from build123d import *

# Parameters (mm, degrees)
SKETCH1_W                      = 150
SKETCH1_H                      = 230
BASE_FLANGE1_DEPTH             = 2
EDGE_FLANGE1_STRIP_W           = 28
EDGE_FLANGE1_STRIP_H           = 2
EDGE_FLANGE1_STRIP_CUT_DEPTH   = 230
EDGE_FLANGE1_STRIP_2_W         = 28
EDGE_FLANGE1_STRIP_2_H         = 2
EDGE_FLANGE1_STRIP_CUT_2_DEPTH = 230
EDGE_FLANGE1_DEPTH             = 230
EDGE_FLANGE1_BEND_DEPTH        = 230
SKETCH15_OUTSIDE_W             = 298.254
SKETCH15_OUTSIDE_H             = 250.254
SKETCH15_OUTSIDE_R             = 8
CUT_EXTRUDE1_DEPTH             = 264.326793168
SKETCH16_R                     = 8
CUT_EXTRUDE2_DEPTH             = 228.055059487
CUT_EXTRUDE3_DEPTH             = 228.055059487
SKETCHED_START                 = 47
SKETCHED_BEND1_DEPTH           = 11.052994728
SKETCHED_BEND1_2_DEPTH         = 11.052994728
CUT_EXTRUDE4_REACH             = 241.866
SKETCH20_R                     = 1.25


# Read off the part's stored shape, not the designer's step: Sketched Bend1
# Sheet-metal steps are written as plain solids
with BuildPart() as part:
    # Sketch1 → Base-Flange1 (new body)
    with BuildSketch(Plane(origin=(0, 0, 0), x_dir=(1, 0, 0), z_dir=(0, 1, 0))):
        Rectangle(SKETCH1_W, SKETCH1_H)
    extrude(amount=-BASE_FLANGE1_DEPTH)

    # Edge-Flange1 strip (across the edge) → Edge-Flange1 strip cut (cut)
    with BuildSketch(Plane(origin=(75, 0, 115), x_dir=(-1, 0, 0), z_dir=(0, 0, -1))):
        with Locations((-4, -1)):
            Rectangle(EDGE_FLANGE1_STRIP_W, EDGE_FLANGE1_STRIP_H)
    extrude(amount=EDGE_FLANGE1_STRIP_CUT_DEPTH, mode=Mode.SUBTRACT)

    # Edge-Flange1 strip 2 (across the edge) → Edge-Flange1 strip cut 2 (cut)
    with BuildSketch(Plane(origin=(-75, 0, -115), x_dir=(1, 0, 0), z_dir=(0, 0, 1))):
        with Locations((-4, -1)):
            Rectangle(EDGE_FLANGE1_STRIP_2_W, EDGE_FLANGE1_STRIP_2_H)
    extrude(amount=EDGE_FLANGE1_STRIP_CUT_2_DEPTH, mode=Mode.SUBTRACT)

    # Edge-Flange1 section (across the edge) → Edge-Flange1 (add)
    with BuildSketch(Plane(origin=(75, 0, 115), x_dir=(-1, 0, 0), z_dir=(0, 0, -1))):
        with BuildLine():
            Line((-2, 10), (-2, 180))
            Line((-2, 180), (0, 180))
            Line((0, 180), (0, 10))
            ThreePointArc((0, 10), (2.928932188, 2.928932188), (10, 0))
            Line((10, 0), (10, -2))
            ThreePointArc((10, -2), (1.514718626, 1.514718626), (-2, 10))
        make_face()
    extrude(amount=EDGE_FLANGE1_DEPTH)

    # Edge-Flange1 section 2 (across the edge) → Edge-Flange1 bend (add)
    with BuildSketch(Plane(origin=(-75, 0, -115), x_dir=(1, 0, 0), z_dir=(0, 0, 1))):
        with BuildLine():
            Line((-2, 10), (-2, 180))
            Line((-2, 180), (0, 180))
            Line((0, 180), (0, 10))
            ThreePointArc((0, 10), (2.928932188, 2.928932188), (10, 0))
            Line((10, 0), (10, -2))
            ThreePointArc((10, -2), (1.514718626, 1.514718626), (-2, 10))
        make_face()
    extrude(amount=EDGE_FLANGE1_BEND_DEPTH)

    # Sketch15 outside → Cut-Extrude1 (cut, through all)
    # profile 1 of 4: a face of its own
    with BuildSketch(Plane.ZY.offset(77)):
        with Locations((0, 89)):
            Rectangle(SKETCH15_OUTSIDE_W, SKETCH15_OUTSIDE_H)
        with BuildLine():
            Line((21.083470393, 171.180744276), (96.507242037, 119.243178795))
            ThreePointArc((96.507242037, 119.243178795), (101.277963521, 113.867184852), (103, 106.888955512))
            Line((103, 106.888955512), (103, 16))
            ThreePointArc((103, 16), (104.757359313, 11.757359313), (109, 10))
            Line((109, 10), (110, 10))
            ThreePointArc((110, 10), (113.535533906, 8.535533906), (115, 5))
            Line((115, 5), (115, -2))
            Line((115, -2), (-115, -2))
            Line((-115, -2), (-115, 99))
            Line((-115, 99), (-115, 150))
            ThreePointArc((-115, 150), (-106.213203436, 171.213203436), (-85, 180))
            Line((-85, 180), (-7.274003064, 180))
            ThreePointArc((-7.274003064, 180), (7.574612801, 177.744304445), (21.083470393, 171.180744276))
        make_face(mode=Mode.SUBTRACT)
    # profile 2 of 4: a face of its own
    with BuildSketch(Plane.ZY.offset(77)):
        with Locations(Location((50, 93, 0), (0, 0, 270))):
            Circle(SKETCH15_OUTSIDE_R)
    # profile 3 of 4: a face of its own
    with BuildSketch(Plane.ZY.offset(77)):
        with Locations(Location((-85, 150, 0), (0, 0, 270))):
            Circle(SKETCH15_OUTSIDE_R)
    # profile 4 of 4: a face of its own
    with BuildSketch(Plane.ZY.offset(77)):
        with Locations(Location((-10, 65, 0), (0, 0, 270))):
            Circle(SKETCH15_OUTSIDE_R)
    extrude(amount=-CUT_EXTRUDE1_DEPTH, mode=Mode.SUBTRACT)

    # Sketch16 → Cut-Extrude2 (cut, through all)
    with BuildSketch(Plane(origin=(0, 0, 0), x_dir=(1, 0, 0), z_dir=(0, 1, 0))):
        with Locations(Location((-42, 39, 0), (0, 0, 270))):
            Circle(SKETCH16_R)
        with Locations(Location((42, 39, 0), (0, 0, 90))):
            Circle(SKETCH16_R)
        with Locations(Location((-42, -31, 0), (0, 0, 90))):
            Circle(SKETCH16_R)
        with Locations(Location((42, -31, 0), (0, 0, 270))):
            Circle(SKETCH16_R)
        with BuildLine():
            Line((7.5, 20), (7.5, -20))
            ThreePointArc((7.5, -20), (0, -27.5), (-7.5, -20))
            Line((-7.5, -20), (-7.5, 20))
            ThreePointArc((-7.5, 20), (0, 27.5), (7.5, 20))
        make_face()
    extrude(amount=-CUT_EXTRUDE2_DEPTH, mode=Mode.SUBTRACT)

    # Sketch18 → Cut-Extrude3 (cut, through all)
    with BuildSketch(Plane(origin=(0, 0, 0), x_dir=(1, 0, 0), z_dir=(0, 1, 0))):
        Polygon((31.4, -45), (44.4, -45), (44.4, -60.052994728), (31.4, -60.052994728), (31.4, -58.052994728), (42.4, -58.052994728), (42.4, -47), (31.4, -47), align=None)
    extrude(amount=-CUT_EXTRUDE3_DEPTH, mode=Mode.SUBTRACT)

    # Sketched Bend1 outline → Sketched Bend1 (cut)
    with BuildSketch(Plane.XY.offset(SKETCHED_START)):
        with BuildLine():
            ThreePointArc((34.035602398, 0), (33.054267209, -1.443395312), (31.4, -2))
            Line((31.4, -2), (42.4, -2))
            Line((42.4, -2), (42.4, 0))
            Line((42.4, 0), (34.035602398, 0))
        make_face()
    extrude(amount=SKETCHED_BEND1_DEPTH, mode=Mode.SUBTRACT)

    # Sketched Bend1 2 outline → Sketched Bend1 2 (add)
    with BuildSketch(Plane.XY.offset(SKETCHED_START)):
        with BuildLine():
            Line((31.4, 0), (34.035602398, 0))
            ThreePointArc((34.035602398, 0), (34.111233029, 0.364854094), (34.1366, 0.7366))
            Line((34.1366, 0.7366), (34.1366, 9.008755099))
            Line((34.1366, 9.008755099), (32.1366, 9.008755099))
            Line((32.1366, 9.008755099), (32.1366, 0.7366))
            ThreePointArc((32.1366, 0.7366), (31.920854855, 0.215745145), (31.4, 0))
        make_face()
    extrude(amount=SKETCHED_BEND1_2_DEPTH)

    # Sketch20 → Cut-Extrude4 (cut, up to next)
    with BuildSketch(Plane.ZY.offset(-32.1366), mode=Mode.PRIVATE) as cut_extrude4_sk1:
        with Locations(Location((52.526497364, 4.9366, 0), (0, 0, 270))):
            Circle(SKETCH20_R)
    cut_extrude4_tool1 = extrude(cut_extrude4_sk1.sketch, amount=-CUT_EXTRUDE4_REACH, mode=Mode.PRIVATE) & part.part
    add(cut_extrude4_tool1.solids().sort_by_distance((32.1366, 4.9366, 52.526497))[0], mode=Mode.SUBTRACT)


solid = part.part
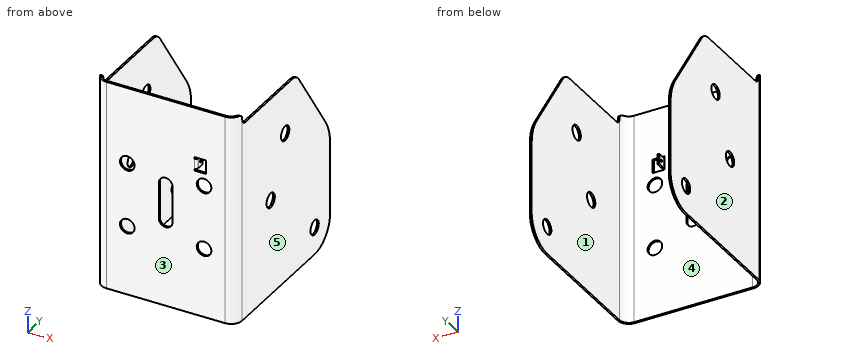
Geometry: final body of the model. Coordinates: model frame, mm. Face numbers are marked on the shaded views. A direction names the side the tool comes from. Coordinates: 2 decimals unless noted, no trailing zeros. Loops run counter-clockwise (first coordinate to the right, second up) from the corner with the lowest first, then second, coordinate; pieces in that order, holes last. Notation, with made-up numbers: (82.25, 59) - (96.25, 59) arc R21 cw to (96.25, 90) - close; hole circle Ø6 at (78, 88). An arc over 180 degrees is marked (long way). One line per question, with ' | ' between items. Start each with the question number.
(1) Cut plane D-D on z = -10. Output: boundary loops of the cut face in (x, y), and give its area (3 significant figures).
(2) First-contact query: pin 1 (1.6 mm diameter, centred on y = -1, z = 50.5, fed in from -X); pin 2 (3 mm diameter, centred on y = 4.94, z = 52.53, fed in from +X); pin 3 (10 mm diameter, centred on x = -53, z = -14, fed in from +Y); pin 4 (21 mm diameter, centred on x = 42, z = -39, fed in from -Y). Flat tips, straight axial feed; report the tip coordinate or a pass-through.
(3) Draft query along X for the marked faces 3, 4 and 5. Return one class per face: +X half, -X half, draft (parallel to the pull), parting line (faces both ways), or undercut.
(4) Cut plane C-C on z = -39. Output: boundary loops of the cut face in (x, y), and give its area (3 significant figures).
(5) Cut plane A-A on x = -42. Output: boundary loops of the cut face in (y, z).
(6) Reachability of the marked faces 1 and 2 from +Z, -Z, +X, -X, +Y, -Y: full face, straight path, thin tool, end or side. Return the list, or none.
(7) Ray query, L1, parallel to X at y = 24, z = 55.5; L2, parallel to X at y = -1, z = 31; L3, parallel to Z at x = -76.05, y = 93. Return the intervals inside material, ascending. Write a range as from..to.
(8) Cut plane B-B on y = 42. Output: boundary loops of the cut face in (x, z).
Here are the results:
1) outline: (-77, 10) arc R12 ccw to (-65, -2) - (-7.5, -2) - (-7.5, 0) - (-65, 0) arc R10 cw to (-75, 10) - (-75, 57) - (-77, 57) - close; (-77, 73) - (-75, 73) - (-75, 180) - (-77, 180) - close; (7.5, -2) - (65, -2) arc R12 ccw to (77, 10) - (77, 57) - (75, 57) - (75, 10) arc R10 cw to (65, 0) - (7.5, 0) - close; (75, 73) - (77, 73) - (77, 180) - (75, 180) - close | area: 915 mm²
2) pin 1: x = -71.32 | pin 2: x = 76.46 | pin 3: y = 0 | pin 4: y = -2
3) face 3: draft | face 4: undercut | face 5: +X half
4) outline: (-77, 10) arc R12 ccw to (-65, -2) - (-50, -2) - (-50, 0) - (-65, 0) arc R10 cw to (-75, 10) - (-75, 180) - (-77, 180) - close; (-34, -2) - (34, -2) - (34, 0) - (-34, 0) - close; (50, -2) - (65, -2) arc R12 ccw to (77, 10) - (77, 180) - (75, 180) - (75, 10) arc R10 cw to (65, 0) - (50, 0) - close | area: 945 mm²
5) outline: (-2, -115) - (0, -115) - (0, -47) - (-2, -47) - close; (-2, -31) - (0, -31) - (0, 23) - (-2, 23) - close; (-2, 39) - (0, 39) - (0, 115) - (-2, 115) - close
6) face 1: +Z, -Z, +Y | face 2: +Z, -Z, -X, +Y, -Y
7) L1: -77..-75, 75..77 | L2: -69.8..-50, -34..34, 50..69.8 | L3: -115..42, 58..103
8) outline: (-77, -115) - (-75, -115) - (-75, 103) - (-77, 103) - close; (75, -115) - (77, -115) - (77, 103) - (75, 103) - close
